```python
from build123d import *

# Parameters (mm, degrees)
BOSS_EXTRUDE1_DEPTH = 35
CUT_EXTRUDE1_REACH  = 79.891
SKETCH4_R           = 1.5
SKETCH4_W           = 7
SKETCH4_H           = 18
SKETCH7_R           = 3.25
CUT_EXTRUDE2_DEPTH  = 3
SKETCH10_R          = 1.35
CUT_EXTRUDE3_DEPTH  = 10
CUT_EXTRUDE4_START  = -10
SKETCH11_R          = 1.35
CUT_EXTRUDE4_DEPTH  = 10
FILLET1_R           = 2.5
FILLET2_R           = 10


with BuildPart() as part:
    # Sketch3 → Boss-Extrude1 (new body)
    with BuildSketch(Plane(origin=(0, 0, 0), x_dir=(1, 0, 0), z_dir=(0, 1, 0))):
        with BuildLine():
            Line((0, 69), (-6, 69))
            Line((-6, 69), (-6, 55))
            add(Edge.make_bspline(
                [(-9, 51), (-9, 55.307083004), (-6, 53.455748632), (-6, 55)],
                knots=[0, 0, 0, 0, 1, 1, 1, 1], degree=3))
            Line((-9, 51), (-9, 35))
            add(Edge.make_bspline(
                [(-9, 35), (-9, 30.102050716), (-6, 31.687720833), (-6, 30)],
                knots=[0, 0, 0, 0, 1, 1, 1, 1], degree=3))
            Line((-6, 30), (-6, 0))
            Line((-6, 0), (0, 0))
            Line((0, 0), (0, 30))
            add(Edge.make_bspline(
                [(-6, 35), (-6, 32.33641875), (0, 33.956398937), (0, 30)],
                knots=[0, 0, 0, 0, 1, 1, 1, 1], degree=3))
            Line((-6, 35), (-6, 51))
            add(Edge.make_bspline(
                [(0, 55), (0, 52.08873611), (-6, 53.842765247), (-6, 51)],
                knots=[0, 0, 0, 0, 1, 1, 1, 1], degree=3))
            Line((0, 55), (0, 69))
        make_face()
    extrude(amount=BOSS_EXTRUDE1_DEPTH)

    # Sketch4 → Cut-Extrude1 (cut, up to next)
    with BuildSketch(Plane.ZY.offset(9), mode=Mode.PRIVATE) as cut_extrude1_sk1:
        with Locations((-4.5, 30.5)):
            Circle(SKETCH4_R)
    cut_extrude1_tool1 = extrude(cut_extrude1_sk1.sketch, amount=-CUT_EXTRUDE1_REACH, mode=Mode.PRIVATE) & part.part
    # Sketch4 → Cut-Extrude1 (cut, up to next)
    with BuildSketch(Plane.ZY.offset(9), mode=Mode.PRIVATE) as cut_extrude1_sk2:
        with Locations((-4.5, 21.5)):
            Circle(SKETCH4_R)
    cut_extrude1_tool2 = extrude(cut_extrude1_sk2.sketch, amount=-CUT_EXTRUDE1_REACH, mode=Mode.PRIVATE) & part.part
    # Sketch4 → Cut-Extrude1 (cut, up to next)
    with BuildSketch(Plane.ZY.offset(9), mode=Mode.PRIVATE) as cut_extrude1_sk3:
        Polygon((-69, 35), (-66, 35), (-69, 0), align=None)
    cut_extrude1_tool3 = extrude(cut_extrude1_sk3.sketch, amount=-CUT_EXTRUDE1_REACH, mode=Mode.PRIVATE) & part.part
    # Sketch4 → Cut-Extrude1 (cut, up to next)
    with BuildSketch(Plane.ZY.offset(9), mode=Mode.PRIVATE) as cut_extrude1_sk4:
        with BuildLine():
            Line((-47.5, 32.25), (-38.5, 32.25))
            ThreePointArc((-38.5, 32.25), (-35.25, 29), (-38.5, 25.75))
            Line((-38.5, 25.75), (-47.5, 25.75))
            ThreePointArc((-47.5, 25.75), (-50.75, 29), (-47.5, 32.25))
        make_face()
    cut_extrude1_tool4 = extrude(cut_extrude1_sk4.sketch, amount=-CUT_EXTRUDE1_REACH, mode=Mode.PRIVATE) & part.part
    # Sketch4 → Cut-Extrude1 (cut, up to next)
    with BuildSketch(Plane.ZY.offset(9), mode=Mode.PRIVATE) as cut_extrude1_sk5:
        with BuildLine():
            Line((-47.5, 22.25), (-38.5, 22.25))
            ThreePointArc((-38.5, 22.25), (-35.25, 19), (-38.5, 15.75))
            Line((-38.5, 15.75), (-47.5, 15.75))
            ThreePointArc((-47.5, 15.75), (-50.75, 19), (-47.5, 22.25))
        make_face()
    cut_extrude1_tool5 = extrude(cut_extrude1_sk5.sketch, amount=-CUT_EXTRUDE1_REACH, mode=Mode.PRIVATE) & part.part
    # Sketch4 → Cut-Extrude1 (cut, up to next)
    with BuildSketch(Plane.ZY.offset(9), mode=Mode.PRIVATE) as cut_extrude1_sk6:
        with BuildLine():
            Line((-47.5, 12.25), (-38.5, 12.25))
            ThreePointArc((-38.5, 12.25), (-35.25, 9), (-38.5, 5.75))
            Line((-38.5, 5.75), (-47.5, 5.75))
            ThreePointArc((-47.5, 5.75), (-50.75, 9), (-47.5, 12.25))
        make_face()
    cut_extrude1_tool6 = extrude(cut_extrude1_sk6.sketch, amount=-CUT_EXTRUDE1_REACH, mode=Mode.PRIVATE) & part.part
    # Sketch4 → Cut-Extrude1 (cut, up to next)
    with BuildSketch(Plane.ZY.offset(9), mode=Mode.PRIVATE) as cut_extrude1_sk7:
        with Locations((-3.5, 9)):
            Rectangle(SKETCH4_W, SKETCH4_H)
    cut_extrude1_tool7 = extrude(cut_extrude1_sk7.sketch, amount=-CUT_EXTRUDE1_REACH, mode=Mode.PRIVATE) & part.part
    # Sketch4 → Cut-Extrude1 (cut, up to next)
    with BuildSketch(Plane.ZY.offset(9), mode=Mode.PRIVATE) as cut_extrude1_sk8:
        with BuildLine():
            Line((-10.75, 20.5), (-10.75, 13))
            ThreePointArc((-10.75, 13), (-17, 6.75), (-23.25, 13))
            Line((-23.25, 13), (-23.25, 20.5))
            ThreePointArc((-23.25, 20.5), (-17, 26.75), (-10.75, 20.5))
        make_face()
    cut_extrude1_tool8 = extrude(cut_extrude1_sk8.sketch, amount=-CUT_EXTRUDE1_REACH, mode=Mode.PRIVATE) & part.part
    add(cut_extrude1_tool1.solids().sort_by_distance((-9, 30.5, -4.5))[0], mode=Mode.SUBTRACT)
    add(cut_extrude1_tool2.solids().sort_by_distance((-9, 21.5, -4.5))[0], mode=Mode.SUBTRACT)
    add(cut_extrude1_tool3.solids().sort_by_distance((-9, 23.333333, -68))[0], mode=Mode.SUBTRACT)
    add(cut_extrude1_tool4.solids().sort_by_distance((-9, 29, -43))[0], mode=Mode.SUBTRACT)
    add(cut_extrude1_tool5.solids().sort_by_distance((-9, 19, -43))[0], mode=Mode.SUBTRACT)
    add(cut_extrude1_tool6.solids().sort_by_distance((-9, 9, -43))[0], mode=Mode.SUBTRACT)
    add(cut_extrude1_tool7.solids().sort_by_distance((-9, 9, -3.5))[0], mode=Mode.SUBTRACT)
    add(cut_extrude1_tool8.solids().sort_by_distance((-9, 16.75, -17))[0], mode=Mode.SUBTRACT)

    # Sketch7 → Cut-Extrude2 (cut)
    with BuildSketch(Plane.ZY.offset(6)):
        with Locations((-4.5, 30.5)):
            Circle(SKETCH7_R)
        with Locations((-4.5, 21.5)):
            Circle(SKETCH7_R)
        with BuildLine():
            Line((-9.3, 20.5), (-9.3, 13))
            ThreePointArc((-9.3, 13), (-17, 5.3), (-24.7, 13))
            Line((-24.7, 13), (-24.7, 20.5))
            ThreePointArc((-24.7, 20.5), (-17, 28.2), (-9.3, 20.5))
        make_face()
    extrude(amount=-CUT_EXTRUDE2_DEPTH, mode=Mode.SUBTRACT)

    # Sketch10 → Cut-Extrude3 (cut)
    with BuildSketch(Plane.XZ):
        with Locations(Location((-3, -59, 0), (0, 0, 270))):
            Circle(SKETCH10_R)
        with Locations(Location((-3, -26, 0), (0, 0, 270))):
            Circle(SKETCH10_R)
    extrude(amount=-CUT_EXTRUDE3_DEPTH, mode=Mode.SUBTRACT)

    # Sketch11 → Cut-Extrude4 (cut)
    with BuildSketch(Plane(origin=(0, 35, 0), x_dir=(1, 0, 0), z_dir=(0, 1, 0)).offset(CUT_EXTRUDE4_START)):
        with Locations(Location((-3, 59, 0), (0, 0, 90))):
            Circle(SKETCH11_R)
    extrude(amount=CUT_EXTRUDE4_DEPTH, mode=Mode.SUBTRACT)

    # Fillet1
    fillet1_edges = [part.edges().sort_by_distance(p)[0] for p in [
        (-3, 0, -69),
        (-3, 35, 0),
        (-3, 35, -66),
        (-3, 18, 0),
        (-3, 18, -7),
    ]]
    fillet(fillet1_edges, radius=FILLET1_R)

    # Fillet2
    fillet2_edges = [part.edges().sort_by_distance(p)[0] for p in [
        (-3, 0, -7),
    ]]
    fillet(fillet2_edges, radius=FILLET2_R)


solid = part.part
```
Read the model definition and answer for the solid it produces. Units are mm, in the model's axes. A direction names the side the tool comes from. Coordinates: 2 decimals unless noted, no trailing zeros. Write each loop counter-clockwise with the first axis right and the second up, starting at its lowest first coordinate (ties: lowest second). Pieces come first, ordered by that corner, then holes. Notation, with made-up numbers: (70, 23.5) -> (99, 23.5) arc R20 cw to (99, 55.5) -> close; hole circle Ø9 at (-13, -34.5). An arc over 180 degrees is marked (long way). Write item = value, one per line.
(1) Section C-C on z = -59 is taken. Write down the section's boundary in (x, y), plus the area to 3 significant figures.
From the geometry:
outline = (-6, 0) -> (-4.35, 0) -> (-4.35, 10) -> (-1.65, 10) -> (-1.65, 0) -> (0, 0) -> (0, 35) -> (-1.65, 35) -> (-1.65, 25) -> (-4.35, 25) -> (-4.35, 35) -> (-6, 35) -> close
area = 156 mm2
(2) Section A-A on z = -21 is taken. Write down the section's boundary in (x, y).
From the geometry:
outline = (-6, 0) -> (0, 0) -> (0, 8.2) -> (-3, 8.2) -> (-3, 6.42) -> (-6, 6.42) -> close; (-6, 27.08) -> (-3, 27.08) -> (-3, 25.3) -> (0, 25.3) -> (0, 35) -> (-6, 35) -> close
(3) Given pin 1 Ø2.5 at (x, y) = (-1, 17.5) entering from +Z; pin 2 Ø2.5 at (x, y) = (-4, 15.5) entering from +Z; pin 3 Ø2.5 at (x, z) = (-3, -59) entering from +Y; pin 4 Ø2.5 at (y, z) = (30.5, -4.5) entering from -X, each flat-ended and moving along its own axis, determine where each tip first touches the part or whether it passes through.
From the geometry:
pin_1 = -0.71
pin_2 = -6.67
pin_3 = 25
pin_4 = through
(4) Straight lines are drawn through the part: L1, parallel to Y at x = -5, z = -4.5; L2, parallel to X at y = 6, z = -59; L3, parallel to Z at x = -2.25, y = 26. For each, find the intervals that lie inside material, in ascending order. Write a range as from..to.
From the geometry:
L1 = 18..18.25, 24.75..27.25, 33.75..35
L2 = -6..-4.35, -1.65..0
L3 = -66.77..-60.12, -57.88..-53.12, -32.75..-19.97, -14.03..0
(5) For a pull along X with two mould halves and no side action, classify faces 4 (the face through (-3.04, 0.79, -68.1)), 5 (the face through (-4.32, 4.93, -58.71)), 6 (the face through (-6, 17, -25)) as +X half, -X half, draft (parallel to the pull), parting line (faces both ways), or undercut.
From the geometry:
face_4 = draft
face_5 = undercut
face_6 = -X half
(6) Which of the six approach directions +Z, -Z, +X, -X, +Y, -Y give full straight-line access (tool end or side, diameter ignored) to faces 1 (the face through (-4.52, 5.3, -16.83)), 2 (the face through (-3, 10, -59)), 3 (the face through (-7.52, 29.07, -35.25))?
From the geometry:
face_1 = -X
face_2 = -Y
face_3 = +X, -X
(7) Section B-B on y = 30.5 is taken. Count the separate pieces of the cut face and the enclosed holes in it, plus the area to 3 significant figures.
From the geometry:
separate_pieces = 3
enclosed_holes = 1
area = 266 mm2
